```python
from build123d import *
from build123d.topology import SkipClean

# Parameters (mm, degrees)
SKETCH1_R           = 1.5
BOSS_EXTRUDE1_DEPTH = 6.3
SKETCH3_R           = 1.9
CUT_EXTRUDE3_DEPTH  = 5.3
BOSS_EXTRUDE2_START = 1.7
BOSS_EXTRUDE2_DEPTH = 1.7
SKETCH7_R           = 4.55
BOSS_EXTRUDE3_DEPTH = 2
SKETCH6_R           = 1.5
SKETCH6_R_2         = 3
CUT_EXTRUDE4_DEPTH  = 22.614925399
CUT_EXTRUDE5_DEPTH  = 22.614925399
BOSS_EXTRUDE4_DEPTH = 3.65


with BuildPart() as part:
    # Sketch1 → Boss-Extrude1 (new body)
    with BuildSketch(Plane(origin=(0, 0, 0), x_dir=(1, 0, 0), z_dir=(0, 1, 0))):
        with BuildLine():
            ThreePointArc((-3.988860539, -11.759062722), (-11.939087297, -11.939087297), (-11.759062722, -3.988860539))
            ThreePointArc((-11.759062722, -3.988860539), (-10, 0), (-11.759062722, 3.988860539))
            ThreePointArc((-11.759062722, 3.988860539), (-11.939087297, 11.939087297), (-3.988860539, 11.759062722))
            ThreePointArc((-3.988860539, 11.759062722), (0, 10), (3.988860539, 11.759062722))
            ThreePointArc((3.988860539, 11.759062722), (11.939087297, 11.939087297), (11.759062722, 3.988860539))
            ThreePointArc((11.759062722, 3.988860539), (10, 0), (11.759062722, -3.988860539))
            ThreePointArc((11.759062722, -3.988860539), (11.939087297, -11.939087297), (3.988860539, -11.759062722))
            ThreePointArc((3.988860539, -11.759062722), (0, -10), (-3.988860539, -11.759062722))
        make_face()
        with Locations(Location((-7.5, 0, 0), (0, 0, 270))):
            Circle(SKETCH1_R, mode=Mode.SUBTRACT)
        with Locations(Location((7.5, 0, 0), (0, 0, 270))):
            Circle(SKETCH1_R, mode=Mode.SUBTRACT)
    extrude(amount=BOSS_EXTRUDE1_DEPTH)

    # Sketch3 → Cut-Extrude3 (cut)
    with BuildSketch(Plane(origin=(0, 6.3, 0), x_dir=(1, 0, 0), z_dir=(0, 1, 0))):
        with Locations(Location((-8.05, 8.05, 0), (0, 0, 270))):
            Circle(SKETCH3_R)
        with Locations(Location((8.05, 8.05, 0), (0, 0, 270))):
            Circle(SKETCH3_R)
        with Locations(Location((8.05, -8.05, 0), (0, 0, 270))):
            Circle(SKETCH3_R)
        with Locations(Location((-8.05, -8.05, 0), (0, 0, 270))):
            Circle(SKETCH3_R)
    extrude(amount=-CUT_EXTRUDE3_DEPTH, mode=Mode.SUBTRACT)

    # Sketch5 → Boss-Extrude2 (add)
    with BuildSketch(Plane(origin=(0, 6.3, 0), x_dir=(1, 0, 0), z_dir=(0, 1, 0)).offset(BOSS_EXTRUDE2_START)):
        with BuildLine():
            Line((-9.5, 6.822197084), (-9.5, -6.822197084))
            ThreePointArc((-9.5, -6.822197084), (-6.706497116, -6.706497116), (-6.822197084, -9.5))
            Line((-6.822197084, -9.5), (6.822197084, -9.5))
            ThreePointArc((6.822197084, -9.5), (6.706497116, -6.706497116), (9.5, -6.822197084))
            Line((9.5, -6.822197084), (9.5, 6.822197084))
            ThreePointArc((9.5, 6.822197084), (6.706497116, 6.706497116), (6.822197084, 9.5))
            Line((6.822197084, 9.5), (-6.822197084, 9.5))
            ThreePointArc((-6.822197084, 9.5), (-6.706497116, 6.706497116), (-9.5, 6.822197084))
        make_face()
    extrude(amount=-BOSS_EXTRUDE2_DEPTH)

    # Sketch7 → Boss-Extrude3 (add)
    with BuildSketch(Plane(origin=(0, 8, 0), x_dir=(1, 0, 0), z_dir=(0, 1, 0))):
        with Locations(Location((0, 0, 0), (0, 0, 270))):
            Circle(SKETCH7_R)
    extrude(amount=BOSS_EXTRUDE3_DEPTH)

    # Sketch6 → Cut-Extrude4 (cut, through all)
    with BuildSketch(Plane(origin=(0, 0, 0), x_dir=(1, 0, 0), z_dir=(0, 1, 0))):
        with Locations(Location((-7.5, 0, 0), (0, 0, 270))):
            Circle(SKETCH6_R)
        with Locations(Location((0, 0, 0), (0, 0, 270))):
            Circle(SKETCH6_R_2)
        with Locations(Location((7.5, 0, 0), (0, 0, 270))):
            Circle(SKETCH6_R)
    extrude(amount=CUT_EXTRUDE4_DEPTH, mode=Mode.SUBTRACT)

    # Sketch8 → Cut-Extrude5 (cut, through all)
    with SkipClean():  # the faces are left unmerged after this step: merging them gives an invalid solid
        with BuildSketch(Plane(origin=(0, 10, 0), x_dir=(1, 0, 0), z_dir=(0, 1, 0))):
            with BuildLine():
                Line((-1.75, 0), (-1.75, 12))
                ThreePointArc((-1.75, 12), (0, 13.75), (1.75, 12))
                Line((1.75, 12), (1.75, 0))
                ThreePointArc((1.75, 0), (0, -1.75), (-1.75, 0))
            make_face()
        extrude(amount=-CUT_EXTRUDE5_DEPTH, mode=Mode.SUBTRACT)

    # Sketch9 → Boss-Extrude4 (add)
    with SkipClean():  # the faces are left unmerged after this step: merging them gives an invalid solid
        with BuildSketch(Plane.XZ):
            with BuildLine():
                Line((-1.75, -2.436698586), (-1.75, 0))
                ThreePointArc((-1.75, 0), (0, 1.75), (1.75, 0))
                Line((1.75, 0), (1.75, -2.436698586))
                ThreePointArc((1.75, -2.436698586), (0, 3), (-1.75, -2.436698586))
            make_face()
        extrude(amount=-BOSS_EXTRUDE4_DEPTH)


solid = part.part
```
Part model, mm, in its own coordinate system. A direction names the side the tool comes from. Give positions to 0.01 mm unless a question says otherwise; leave off trailing zeros. Write each loop counter-clockwise with the first axis right and the second up, starting at its lowest first coordinate (ties: lowest second). Pieces come first, ordered by that corner, then holes. Notation, with made-up numbers: M -16.5,65.5 L -1.5,65.5 A31 ccw -1.5,98.5 Z; hole C -5.75,-20.5 d7. An arc over 180 degrees is marked long. Use CSV: the item, a comma, the result in double quotes.
Item 1: Slice it at A-A on y = 2.75. Write the cut outline in (x, z), plus the area to 3 significant figures.
Taken from the geometry:
outline,"M -11.76,-3.99 A5.5 ccw long -3.99,-11.76 A5.4 cw -1.75,-10.29 L -1.75,0 A1.75 cw 1.75,0 L 1.75,-10.29 A5.4 cw 3.99,-11.76 A5.5 ccw long 11.76,-3.99 A5.4 cw 11.76,3.99 A5.5 ccw long 3.99,11.76 A5.4 cw -3.99,11.76 A5.5 ccw long -11.76,3.99 A5.4 cw Z; hole C -8.05,-8.05 d3.8; hole C -8.05,8.05 d3.8; hole C -7.5,0 d3; hole C 7.5,0 d3; hole C 8.05,-8.05 d3.8; hole C 8.05,8.05 d3.8"
area,"495 mm²"
Item 2: Pull direction X, two halves, no side cores. Call faces 5 (the face through (-0.175, 8.986, 4.547)), 6 (the face through (0, 7, 3)), 7 (the face through (3, 0, 0)): +X half, -X half, draft (parallel to the pull), parting line (faces both ways), or undercut.
Taken from the geometry:
face 5,"parting line"
face 6,"undercut"
face 7,"draft"
Item 3: Slice it at C-C on y = 7.25. Write the cut outline in (x, z).
Taken from the geometry:
outline,"M -9.5,-6.82 A1.9 cw long -6.82,-9.5 L -1.75,-9.5 L -1.75,-2.44 A3 cw long 1.75,-2.44 L 1.75,-9.5 L 6.82,-9.5 A1.9 cw long 9.5,-6.82 L 9.5,6.82 A1.9 cw long 6.82,9.5 L -6.82,9.5 A1.9 cw long -9.5,6.82 Z; hole C -7.5,0 d3; hole C 7.5,0 d3"
Item 4: Slice it at B-B on z = -8.05. Write the cut outline in (x, y), plus the area to 3 significant figures.
Taken from the geometry:
outline,"M -13.55,0 L -1.75,0 L -1.75,8 L -6.15,8 L -6.15,1 L -9.95,1 L -9.95,6.3 L -13.55,6.3 Z; M 1.75,0 L 13.55,0 L 13.55,6.3 L 9.95,6.3 L 9.95,1 L 6.15,1 L 6.15,8 L 1.75,8 Z"
area,"123 mm²"
Item 5: Drill centre lines: probe 1 along X at (y, z) = (4, -8); probe 2 along X at (y, z) = (5.1, 8.05); probe 3 along Z at (x, y) = (8.05, 4.6). Where is each one in solid material? Low to high.
Taken from the geometry:
probe 1,"x = -13.55 to -9.95, -6.15 to -1.75, 1.75 to 6.15, 9.95 to 13.55"
probe 2,"x = -13.55 to -9.95, -6.15 to 6.15, 9.95 to 13.55"
probe 3,"z = -13.55 to -9.95, -6.15 to -1.4, 1.4 to 6.15, 9.95 to 13.55"
Item 6: Which spindle directions (+Z, -Z, +X, -X, +Y, -Y) get a long thin tool onto all of the face, cutting with end or side? Do faces 1 (the face through (-9.5, 7, 0)), 2 (the face through (4, 7, -9.5)), 3 (the face through (-8, 1, -8)), 4 (the face through (-10, 3, 0)). Say none if no direction does.
Taken from the geometry:
face 1,"+Z, -Z, -X, +Y"
face 2,"-Z, +X, -X, +Y"
face 3,"+Y"
face 4,"-X, +Y, -Y"
Item 7: Slice it at D-D on x = -10.5. Write the cut outline in (y, z).
Taken from the geometry:
outline,"M 0,-12.97 L 6.3,-12.97 L 6.3,-2.27 L 0,-2.27 Z; M 0,2.27 L 6.3,2.27 L 6.3,12.97 L 0,12.97 Z"
Item 8: Pin check, flat tips, straight feed: P1, Ø1.9, axis at x = 8, z = 7.5, coming from the +Y side; P2, Ø5, axis at y = 4.5, z = 1, coming from the +X side; P3, Ø6, axis at x = -9.5, z = 4, coming from the +Y side. Stop position of each tip, or through.
Taken from the geometry:
P1,"stops at y = 1"
P2,"stops at x = 11.29"
P3,"stops at y = 8"
